from build123d import *

# Parameters (mm, degrees)
F0_R     = 1.5875
F1_DEPTH = 3.175
F2_DEPTH = 2.54


with BuildPart() as f1:
    # F0 (on Top) → F1 (new body)
    with BuildSketch(Plane.XY):
        with BuildLine():
            Line((48.41875, 12.47476), (-0.595312, 3.11869))
            ThreePointArc((-0.595312, 3.11869), (-3.175, 0), (-0.595312, -3.11869))
            Line((-0.595312, -3.11869), (48.41875, -12.47476))
            ThreePointArc((48.41875, -12.47476), (63.5, 0), (48.41875, 12.47476))
        make_face()
        Circle(F0_R, mode=Mode.SUBTRACT)
        Circle(F0_R)
    extrude(amount=F1_DEPTH)

    # F0 (on Top) → F2 (join)
    with BuildSketch(Plane.XY):
        Circle(F0_R)
    extrude(amount=-F2_DEPTH)


solid = f1.part
Check sheet for the modelled part. Datum: model origin and axes. Units: mm. A direction names the side the tool comes from. Round coordinates to 2 decimals unless told otherwise and drop trailing zeros. Loops run counter-clockwise (first coordinate to the right, second up) from the corner with the lowest first, then second, coordinate; pieces in that order, holes last.
1. Sectioned sample at A-A on y = 0. Record the boundary of the cut face in (x, z) (1 decimal), and give its area (3 significant figures).
2. Sectioned sample at C-C on x = 50.8. Record the boundary of the cut face in (y, z) (3 decimals), and give its area (3 significant figures).
3. Gauge pin test, flat ends, axial feed: pin 1 Ø2 at (x, z) = (20, 1) entering from -Y; pin 2 Ø3 at (x, y) = (12.5, -0.5) entering from -Z. Record the tip position at first contact, or that the pin passes through.
4. Set-up check for faces 1 (the flat face through (37, 0, 3.175)), 2 (the cylindrical face through (-0.34, -1.55, -1.25)): record each of +Z, -Z, +X, -X, +Y, -Y from which the full face is reachable in a straight line by a thin tool's end or side.
5. Sectioned sample at D-D on x = 0. Record the boundary of the cut face in (y, z) (1 decimal).
6. Scan lines: probe 1 along Z at (x, y) = (52, 4) (3 decimals); probe 2 along Y at (x, z) = (11.5, 0.15); probe 3 along X at (y, z) = (-0.5, 1). Record each from-to range of solid material in increasing order.
7. Sectioned sample at B-B on z = 0.95. Record the boundary of the cut face in (x, y) (3 decimals).
Recorded:
1. outline: (-3.2, 0) - (-1.6, 0) - (-1.6, -2.5) - (1.6, -2.5) - (1.6, 0) - (63.5, 0) - (63.5, 3.2) - (-3.2, 3.2) - close
1. area: 220 mm2
2. outline: (-12.7, 0) - (12.7, 0) - (12.7, 3.175) - (-12.7, 3.175) - close
2. area: 80.6 mm2
3. pin 1: stops at y = -7.24
3. pin 2: stops at z = 0
4. face 1: +Z, +X, -X, +Y, -Y
4. face 2: -Z
5. outline: (-3.2, 0) - (-1.6, 0) - (-1.6, -2.5) - (1.6, -2.5) - (1.6, 0) - (3.2, 0) - (3.2, 3.2) - (-3.2, 3.2) - close
6. probe 1: z = 0 to 3.175
6. probe 2: y = -5.43 to 5.43
6. probe 3: x = -3.14 to 63.49
7. outline: (-0.595, -3.119) - (48.419, -12.475) arc R12.7 ccw (long way) to (48.419, 12.475) - (-0.595, 3.119) arc R3.175 ccw to start
